The listing builds one solid part. Answer for the finished solid, in the listing's coordinates (mm). Round coordinates to 2 decimals unless told otherwise and drop trailing zeros. Loops run counter-clockwise (first coordinate to the right, second up) from the corner with the lowest first, then second, coordinate; pieces in that order, holes last. Notation, with made-up numbers: (26.25, 11.25) -> (65.25, 11.25) arc R22 ccw to (65.25, 23.25) -> close; hole circle Ø1 at (-25.75, 42). An arc over 180 degrees is marked (long way). Use a Markdown table: item, result. Add a question column.
Q1. Section B-B on y = -1.1 is taken. Give the vertices of the cut face in (x, z).
Q2. Section A-A on z = 14 is taken. Give the vertices of the cut face in (x, y), then the cut area to 3 significant figures.
Q3. Section D-D on x = 6 is taken. Give the vertices of the cut face in (y, z).
Q4. Consider line 1 (X direction, y = -1, z = 13); line 2 (X direction, y = -0.85, z = 18); line 3 (X direction, y = -1.05, z = 23.5). Determine where each line is inside the solid, lowest interval first.
Q5. Given pin 1 Ø0.6 at (x, y) = (8.5, -1.5) entering from +Z; pin 2 Ø0.6 at (x, y) = (-28, -1.5) entering from +Z; pin 3 Ø1 at (x, y) = (-27.5, -0.5) entering from -Z, each flat-ended and moving along its own axis, determine where each tip first touches the part or whether it passes through.
Q6. Section C-C on x = -6.5 is taken. Give the vertices of the cut face in (y, z).
from build123d import *

# Parameters (mm, degrees)
F0_W      = 91
F0_H      = 35
F1_DEPTH  = 2
F2_W      = 15
F2_H      = 12
F3_DEPTH  = 3
F5_DEPTH  = 5
F6_W      = 57
F6_H      = 3
F7_DEPTH  = 3
F8_W      = 3
F8_H      = 5
F9_DEPTH  = 9
F10_W     = 3
F10_H     = 6.3
F11_DEPTH = 4
F12_R     = 2
F13_DEPTH = 4
F14_W     = 6
F14_H     = 4
F15_DEPTH = 4


with BuildPart() as f1:
    # F0 (on Front) → F1 (new body)
    with BuildSketch(Plane.XZ):
        with Locations((-18.235627, 10.280461)):
            Rectangle(F0_W, F0_H)
    extrude(amount=F1_DEPTH)

    # F2 (on Front) → F3 (cut)
    with BuildSketch(Plane.XZ):
        with Locations((7.5, 21.966114)):
            Rectangle(F2_W, F2_H)
    extrude(amount=F3_DEPTH, mode=Mode.SUBTRACT)

    # F4 (on Front) → F5 (cut)
    with BuildSketch(Plane.XZ):
        Polygon((-65.685175, 18.899074), (0, 18.899074), (0, 18.929425), (0, 28.964864), (-65.685175, 28.964864), align=None)
    extrude(amount=F5_DEPTH, mode=Mode.SUBTRACT)

    # F6 (on Front) → F7 (cut)
    with BuildSketch(Plane.XZ):
        with Locations((-31.5, 17.516951)):
            Rectangle(F6_W, F6_H)
    extrude(amount=F7_DEPTH, mode=Mode.SUBTRACT)

    # F8 (on Front) → F9 (cut)
    with BuildSketch(Plane.XZ):
        with Locations((-27.711618, 13.540782)):
            Rectangle(F8_W, F8_H)
    extrude(amount=F9_DEPTH, mode=Mode.SUBTRACT)

    # F10 (on Front) → F11 (cut)
    with BuildSketch(Plane.XZ):
        with Locations((-27.678377, -4.335782)):
            Rectangle(F10_W, F10_H)
    extrude(amount=F11_DEPTH, mode=Mode.SUBTRACT)

    # F12 (on Front) → F13 (cut)
    with BuildSketch(Plane.XZ):
        with Locations((-27.586486, 5.011399)):
            Circle(F12_R)
    extrude(amount=F13_DEPTH, mode=Mode.SUBTRACT)

    # F14 (on Front) → F15 (cut)
    with BuildSketch(Plane.XZ):
        with Locations((22.072674, 24.467368)):
            Rectangle(F14_W, F14_H)
    extrude(amount=F15_DEPTH, mode=Mode.SUBTRACT)


solid = f1.part
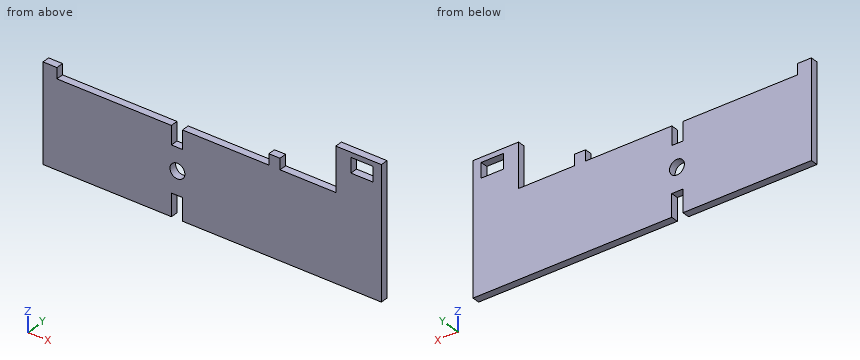
Checked values:
| question | item | result |
|---|---|---|
| 1 | outline | (-63.74, -7.22) -> (-29.18, -7.22) -> (-29.18, -1.19) -> (-26.18, -1.19) -> (-26.18, -7.22) -> (27.26, -7.22) -> (27.26, 27.78) -> (15, 27.78) -> (15, 15.97) -> (0, 15.97) -> (0, 18.9) -> (-3, 18.9) -> (-3, 16.02) -> (-26.21, 16.02) -> (-26.21, 11.04) -> (-29.21, 11.04) -> (-29.21, 16.02) -> (-60, 16.02) -> (-60, 18.9) -> (-63.74, 18.9) -> close; hole circle Ø4 at (-27.59, 5.01); hole (19.07, 22.47) -> (25.07, 22.47) -> (25.07, 26.47) -> (19.07, 26.47) -> close |
| 2 | outline | (-63.74, -2) -> (-29.21, -2) -> (-29.21, 0) -> (-63.74, 0) -> close; (-26.21, -2) -> (27.26, -2) -> (27.26, 0) -> (-26.21, 0) -> close |
| 2 | area | 176 mm2 |
| 3 | outline | (-2, -7.22) -> (0, -7.22) -> (0, 15.97) -> (-2, 15.97) -> close |
| 4 | line 1 | x = -63.74 to -29.21, -26.21 to 27.26 |
| 4 | line 2 | x = -63.74 to -60, -3 to 0, 15 to 27.26 |
| 4 | line 3 | x = 15 to 19.07, 25.07 to 27.26 |
| 5 | pin 1 | stops at z = 15.97 |
| 5 | pin 2 | stops at z = 11.04 |
| 5 | pin 3 | stops at z = -1.19 |
| 6 | outline | (-2, -7.22) -> (0, -7.22) -> (0, 16.02) -> (-2, 16.02) -> close |
